Read the model definition and answer for the solid it produces. Units are mm, in the model's axes. A direction names the side the tool comes from. Round coordinates to 2 decimals unless told otherwise and drop trailing zeros. Write each loop counter-clockwise with the first axis right and the second up, starting at its lowest first coordinate (ties: lowest second). Pieces come first, ordered by that corner, then holes. Notation, with made-up numbers: (0.25, 38) - (24.25, 38) arc R23 cw to (24.25, 46) - close; hole circle Ø10 at (53, 22.25). An arc over 180 degrees is marked (long way). Use one line per item in the form item = value. Start each with the question number.
1) The part is cut by section B-B, the plane x = -4. Give the vertices of the cut face in (y, z).
2) The part is cut by section A-A, the plane y = 8. Give the vertices of the cut face in (x, z), plus the area to 3 significant figures.
3) For faces 1 (the face through (11, 30, -13)), 2 (the face through (11, 0, -13)), 3 (the face through (11, 0, 13)), 4 (the face through (11, 30, 13)), determine the directions among +Z, -Z, +X, -X, +Y, -Y from which every point of the face is accessible in a straight line to the end or side of a thin tool.
4) Consider line 1 along Z through (x, y) = (-20.5, 38.5); line 2 along Y through (x, z) = (13.5, 14). Determine where each line is inside the solid, lowest interval first. Write a range as from..to.
5) Each of these flat-tipped pins is pushed along its axis until it touches: pin 1 (15 mm diameter, centred on x = -5, y = 24, fed in from -Z); pin 2 (3 mm diameter, centred on x = -12, z = -13, fed in from -Y); pin 3 (4 mm diameter, centred on x = -15.5, y = 22, fed in from +Z); pin 4 (8 mm diameter, centred on x = 9, z = 14.5, fed in from -Y). Where does it stop, or does it pass through?
6) The part is cut by section D-D, the plane x = 8.5. Give the vertices of the cut face in (y, z).
7) The part is cut by section C-C, the plane z = 12.5. Give the vertices of the cut face in (x, y).
from build123d import *

# Parameters (mm, degrees)
SKETCH1_W           = 60
SKETCH1_H           = 50
BOSS_EXTRUDE1_DEPTH = 10
REVOLVE1_DEPTH      = 30


# Read off the part's stored shape, not the designer's step: Revolve1
with BuildPart() as part:
    # Sketch1 → Boss-Extrude1 (new, symmetric)
    with BuildSketch(Plane.XY):
        with Locations((0, 15)):
            Rectangle(SKETCH1_W, SKETCH1_H)
    extrude(amount=BOSS_EXTRUDE1_DEPTH, both=True)

    # Revolve1 outline → Revolve1 (add)
    with BuildSketch(Plane(origin=(0, 0, 0), x_dir=(1, 0, 0), z_dir=(0, 1, 0))):
        with BuildLine():
            Line((10, 17.320508076), (5.773502692, 10))
            Line((5.773502692, 10), (17.320508076, 10))
            ThreePointArc((17.320508076, 10), (14.142135624, 14.142135624), (10, 17.320508076))
        make_face()
        with BuildLine():
            ThreePointArc((10, -17.320508076), (14.142135624, -14.142135624), (17.320508076, -10))
            Line((17.320508076, -10), (5.773502692, -10))
            Line((5.773502692, -10), (10, -17.320508076))
        make_face()
    extrude(amount=REVOLVE1_DEPTH)


solid = part.part
Geometry results:
q1.outline = (-10, -10) - (40, -10) - (40, 10) - (-10, 10) - close
q2.outline = (-30, -10) - (5.77, -10) - (10, -17.32) arc R20 ccw to (17.32, -10) - (30, -10) - (30, 10) - (17.32, 10) arc R20 ccw to (10, 17.32) - (5.77, 10) - (-30, 10) - close
q2.area = 1,290 mm2
q3.face_1 = -Z, +X, -X, +Y
q3.face_2 = -Z, +X, -X, -Y
q3.face_3 = +Z, +X, -X, -Y
q3.face_4 = +Z, +X, -X, +Y
q4.line_1 = -10..10
q4.line_2 = 0..30
q5.pin_1 = -10
q5.pin_2 = through
q5.pin_3 = 10
q5.pin_4 = 0
q6.outline = (-10, -10) - (0, -10) - (0, -14.72) - (30, -14.72) - (30, -10) - (40, -10) - (40, 10) - (30, 10) - (30, 14.72) - (0, 14.72) - (0, 10) - (-10, 10) - close
q7.outline = (7.22, 0) - (15.61, 0) - (15.61, 30) - (7.22, 30) - close
